Part model, mm, in its own coordinate system. A direction names the side the tool comes from. Round coordinates to 2 decimals unless told otherwise and drop trailing zeros. Write each loop counter-clockwise with the first axis right and the second up, starting at its lowest first coordinate (ties: lowest second). Pieces come first, ordered by that corner, then holes. Notation, with made-up numbers: M -21.5,-20 L 30.5,-20 A16 cw 30.5,-9 Z; hole C 14.5,50 d6. An arc over 180 degrees is marked long. Use a Markdown table: item, result. Add a question column.
1) Two-plate mould, pull along Y, no slides. Class faces 1 (the face through (0, 0, 0)), 2 (the face through (19, 9, -4.5)), 3 (the face through (-16.175, 21.435, 0.43)): released by +Y, released by -Y, zero draft, split by the parting line, or undercut.
2) Slice it at B-B on z = 0. Write the cut outline in (x, y), plus the area to 3 significant figures.
3) Wall check: probe 1 along X at (y, z) = (21.4, 0); probe 2 along Z at (x, y) = (16.85, 20.75); probe 3 along X at (y, z) = (12.25, 2.25). Give the ranges that are in metal, low to high.
4) Slice it at C-C on y = 9.5. Write the cut outline in (x, z), plus the area to 3 significant figures.
5) Slice it at A-A on y = 6.25. Write the cut outline in (x, z), plus the area to 3 significant figures.
6) Which spindle directions (+Z, -Z, +X, -X, +Y, -Y) get a long thin tool onto all of the face, cutting with end or side? Do faces 4 (the face through (23.25, 14, 0)), 5 (the face through (17, 18.9, 0)), 6 (the face through (19, 14, -9)), 7 (the face through (15.25, 14, 0)), 8 (the face through (19, 14, 9)). Say none if no direction does.
7) Slice it at D-D on x = -16.85. Write the cut outline in (y, z).
8) Drop flat-ended pins along their axis: P1, Ø6, axis at x = 18.5, y = 11.5, coming from the +Z side; P2, Ø1.5, axis at x = 17.5, y = 9, coming from the -Z side; P3, Ø1.4, axis at x = 16.85, z = 0, coming from the +Y side. Give the stop position or say it passes through.
```python
from build123d import *

# Parameters (mm, degrees)
SKETCH1_W           = 54
SKETCH1_H           = 28
BOSS_EXTRUDE1_DEPTH = 4
SKETCH4_W           = 8
SKETCH4_H           = 18
BOSS_EXTRUDE3_DEPTH = 19.9
FILLET1_R           = 5
SKETCH5_R           = 0.8
CUT_EXTRUDE1_DEPTH  = 5
SKETCH6_W           = 9
SKETCH6_H           = 5
CUT_EXTRUDE2_DEPTH  = 13
FILLET4_R           = 0.5
FILLET5_R           = 0.5


with BuildPart() as part:
    # Sketch1 → Boss-Extrude1 (new body)
    with BuildSketch(Plane(origin=(0, 0, 0), x_dir=(1, 0, 0), z_dir=(0, 1, 0))):
        Rectangle(SKETCH1_W, SKETCH1_H)
    extrude(amount=BOSS_EXTRUDE1_DEPTH)

    # Sketch4 → Boss-Extrude3 (add)
    with BuildSketch(Plane(origin=(0, 4, 0), x_dir=(1, 0, 0), z_dir=(0, 1, 0))):
        with Locations((-19.25, 0)):
            Rectangle(SKETCH4_W, SKETCH4_H)
    boss_extrude3 = extrude(amount=BOSS_EXTRUDE3_DEPTH)

    # Mirror2: Boss-Extrude3 across plane
    add(boss_extrude3.mirror(Plane(origin=(0, 0, 0), x_dir=(0, 0, 1), z_dir=(1, 0, 0))))

    # Fillet1
    fillet1_edges = [part.edges().sort_by_distance(p)[0] for p in [
        (27, 2, 14),
        (-27, 2, 14),
        (-27, 2, -14),
        (27, 2, -14),
    ]]
    fillet(fillet1_edges, radius=FILLET1_R)

    # Sketch5 → Cut-Extrude1 (cut)
    with BuildSketch(Plane(origin=(0, 23.9, 0), x_dir=(1, 0, 0), z_dir=(0, 1, 0))):
        with Locations(Location((-16.85, 0, 0), (0, 0, 270))):
            Circle(SKETCH5_R)
    cut_extrude1 = extrude(amount=-CUT_EXTRUDE1_DEPTH, mode=Mode.SUBTRACT)

    # Mirror3: Cut-Extrude1 across plane
    add(cut_extrude1.mirror(Plane(origin=(0, 0, 0), x_dir=(0, 0, 1), z_dir=(1, 0, 0))), mode=Mode.SUBTRACT)

    # Sketch6 → Cut-Extrude2 (cut)
    with BuildSketch(Plane(origin=(23.25, 0, 0), x_dir=(0, 0, -1), z_dir=(1, 0, 0))):
        with Locations((0, 9.492209163)):
            Rectangle(SKETCH6_W, SKETCH6_H)
    extrude(amount=-CUT_EXTRUDE2_DEPTH, mode=Mode.SUBTRACT)

    # Fillet4
    fillet4_edges = [part.edges().sort_by_distance(p)[0] for p in [
        (-19.25, 23.9, -9),
        (-23.25, 23.9, 0),
        (-19.25, 23.9, 9),
        (19.25, 23.9, 9),
        (23.25, 23.9, 0),
        (19.25, 23.9, -9),
    ]]
    fillet(fillet4_edges, radius=FILLET4_R)

    # Fillet5
    # the kernel refuses this fillet: 0.5 mm, written as the material it takes off along each edge
    with BuildSketch(Plane(origin=(-22.75, 23.4, 8.5), x_dir=(-1, 0, 0), z_dir=(0, 0, 1))) as fillet5_piece_1_section:
        Polygon((0, 0), (FILLET5_R, 0), (FILLET5_R, -FILLET5_R), (0, -FILLET5_R), align=None)
    fillet5_piece_1 = extrude(amount=FILLET5_R, mode=Mode.PRIVATE)
    fillet5_piece_1 = fillet5_piece_1 - Plane(origin=(-22.75, 23.4, 8.5), x_dir=(0.7071067811865475, -0.7071067811865475, 0), z_dir=(0, 0, 1)) * Sphere(FILLET5_R, mode=Mode.PRIVATE)
    add(fillet5_piece_1, mode=Mode.SUBTRACT)
    with BuildSketch(Plane(origin=(-22.75, 23.4, -8.5), x_dir=(-1, 0, 0), z_dir=(0, 0, -1))) as fillet5_piece_2_section:
        Polygon((0, 0), (FILLET5_R, 0), (FILLET5_R, FILLET5_R), (0, FILLET5_R), align=None)
    fillet5_piece_2 = extrude(amount=FILLET5_R, mode=Mode.PRIVATE)
    fillet5_piece_2 = fillet5_piece_2 - Plane(origin=(-22.75, 23.4, -8.5), x_dir=(0.7071067811865475, -0.7071067811865475, 0), z_dir=(0, 0, -1)) * Sphere(FILLET5_R, mode=Mode.PRIVATE)
    add(fillet5_piece_2, mode=Mode.SUBTRACT)
    with BuildSketch(Plane(origin=(22.75, 23.4, -8.5), x_dir=(1, 0, 0), z_dir=(0, 0, -1))) as fillet5_piece_3_section:
        Polygon((0, 0), (FILLET5_R, 0), (FILLET5_R, -FILLET5_R), (0, -FILLET5_R), align=None)
    fillet5_piece_3 = extrude(amount=FILLET5_R, mode=Mode.PRIVATE)
    fillet5_piece_3 = fillet5_piece_3 - Plane(origin=(22.75, 23.4, -8.5), x_dir=(-0.7071067811865475, -0.7071067811865475, 0), z_dir=(0, 0, -1)) * Sphere(FILLET5_R, mode=Mode.PRIVATE)
    add(fillet5_piece_3, mode=Mode.SUBTRACT)
    with BuildSketch(Plane(origin=(22.75, 23.4, 8.5), x_dir=(0, 0, 1), z_dir=(1, 0, 0))) as fillet5_piece_4_section:
        Polygon((0, 0), (FILLET5_R, 0), (FILLET5_R, -FILLET5_R), (0, -FILLET5_R), align=None)
    fillet5_piece_4 = extrude(amount=FILLET5_R, mode=Mode.PRIVATE)
    fillet5_piece_4 = fillet5_piece_4 - Plane(origin=(22.75, 23.4, 8.5), x_dir=(0, -0.7071067811865475, -0.7071067811865475), z_dir=(1, 0, 0)) * Sphere(FILLET5_R, mode=Mode.PRIVATE)
    add(fillet5_piece_4, mode=Mode.SUBTRACT)
    with BuildSketch(Plane(origin=(-23.25, 4, -9), x_dir=(1, 0, 0), z_dir=(0, 1, 0))) as fillet5_piece_5:
        with BuildLine():
            CenterArc((FILLET5_R, -FILLET5_R), FILLET5_R, 90, 90)
            Line((0, -FILLET5_R), (0, 0))
            Line((0, 0), (FILLET5_R, 0))
        make_face()
    extrude(amount=19.4, mode=Mode.SUBTRACT)
    with BuildSketch(Plane(origin=(-23.25, 4, 9), x_dir=(1, 0, 0), z_dir=(0, 1, 0)), Plane(origin=(23.25, 4, 9), x_dir=(0, 0, -1), z_dir=(0, 1, 0)), Plane(origin=(23.25, 4, -9), x_dir=(-1, 0, 0), z_dir=(0, 1, 0))) as fillet5_piece_6:
        with BuildLine():
            CenterArc((FILLET5_R, FILLET5_R), FILLET5_R, 180, 90)
            Line((0, FILLET5_R), (0, 0))
            Line((0, 0), (FILLET5_R, 0))
        make_face()
    extrude(amount=19.4, mode=Mode.SUBTRACT)


solid = part.part
```
Entries:
| question | item | result |
|---|---|---|
| 1 | face 1 | released by -Y |
| 1 | face 2 | undercut |
| 1 | face 3 | zero draft |
| 2 | outline | M -27,0 L 27,0 L 27,4 L 23.25,4 L 23.25,6.99 L 15.25,6.99 L 15.25,4 L -15.25,4 L -15.25,23.9 L -16.05,23.9 L -16.05,18.9 L -17.65,18.9 L -17.65,23.9 L -22.75,23.9 A0.5 ccw -23.25,23.4 L -23.25,4 L -27,4 Z; M 15.25,11.99 L 23.25,11.99 L 23.25,23.4 A0.5 ccw 22.75,23.9 L 17.65,23.9 L 17.65,18.9 L 16.05,18.9 L 16.05,23.9 L 15.25,23.9 Z |
| 2 | area | 478 mm^2 |
| 3 | probe 1 | x = -23.25 to -17.65, -16.05 to -15.25, 15.25 to 16.05, 17.65 to 23.25 |
| 3 | probe 2 | z = -9 to -0.8, 0.8 to 9 |
| 3 | probe 3 | x = -23.25 to -15.25, 15.25 to 23.25 |
| 4 | outline | M -23.25,-8.5 A0.5 ccw -22.75,-9 L -15.25,-9 L -15.25,9 L -22.75,9 A0.5 ccw -23.25,8.5 Z; M 15.25,-9 L 22.75,-9 A0.5 ccw 23.25,-8.5 L 23.25,-4.5 L 15.25,-4.5 Z; M 15.25,4.5 L 23.25,4.5 L 23.25,8.5 A0.5 ccw 22.75,9 L 15.25,9 Z |
| 4 | area | 216 mm^2 |
| 5 | outline | M -23.25,-8.5 A0.5 ccw -22.75,-9 L -15.25,-9 L -15.25,9 L -22.75,9 A0.5 ccw -23.25,8.5 Z; M 15.25,-9 L 22.75,-9 A0.5 ccw 23.25,-8.5 L 23.25,8.5 A0.5 ccw 22.75,9 L 15.25,9 Z |
| 5 | area | 288 mm^2 |
| 6 | face 4 | +Z, -Z, +X, +Y |
| 6 | face 5 | +Y |
| 6 | face 6 | -Z, +X, -X, +Y |
| 6 | face 7 | +Z, -Z, +Y |
| 6 | face 8 | +Z, +X, -X, +Y |
| 7 | outline | M 0,-14 L 4,-14 L 4,-9 L 23.4,-9 A0.5 ccw 23.9,-8.5 L 23.9,-0.8 L 18.9,-0.8 L 18.9,0.8 L 23.9,0.8 L 23.9,8.5 A0.5 ccw 23.4,9 L 4,9 L 4,14 L 0,14 Z |
| 8 | P1 | stops at z = 9 |
| 8 | P2 | stops at z = -9 |
| 8 | P3 | stops at y = 18.9 |
